The figure shows three views and two pictorial views of one solid part (mm, origin at its lowest corner). Answer the questions. Coordinates: 2 decimals unless noted, no trailing zeros. Write each loop counter-clockwise with the first axis right and the second up, starting at its lowest first coordinate (ties: lowest second). Pieces come first, ordered by that corner, then holes.
Item 1: Section C-C (z = 12.25) is taken. Give the vertices of the cut face in (x, y).
Item 2: Section A-A (y = 0.2) is taken. Give the vertices of the cut face in (x, z), then the cut area to 3 significant figures.
Item 3: Section B-B (x = 8) is taken. Give the vertices of the cut face in (y, z).
Item 4: This flat-tipped pin is pushed along its axis until it touches: P1, Ø3, axis at x = 3, z = 2, coming from the -Y side. Where does it stop, or does it pass through?
Item 5: Straight lines are drawn through the part: probe 1 along X at (y, z) = (0.45, 7.5) (1 decimal); probe 2 along Z at (x, y) = (8, 0.3); probe 3 along Z at (x, y) = (5.5, 0.3). For each, find the intervals that lie inside material, in ascending order.
Item 6: Section D-D (x = 2) is taken. Give the vertices of the cut face in (y, z), then the cut area to 3 significant figures.
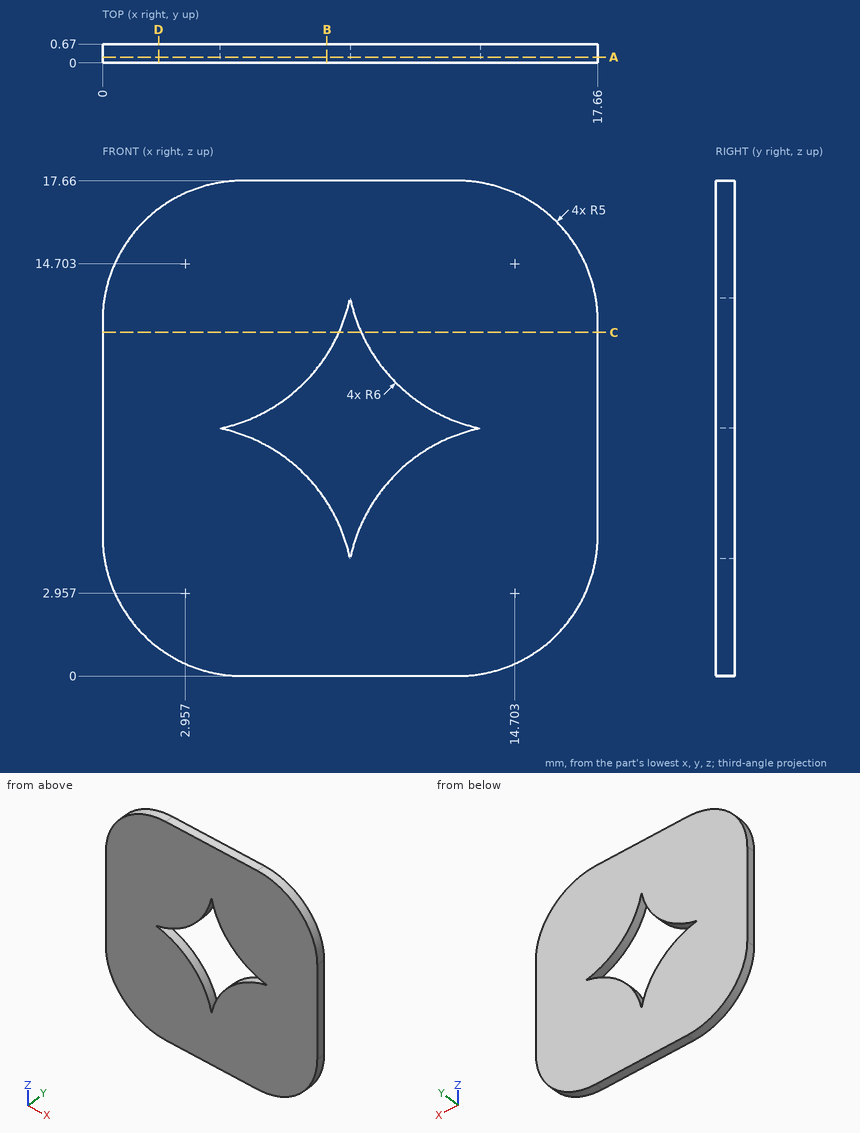
Established:
1. outline: (0, 0) - (8.43, 0) - (8.43, 0.67) - (0, 0.67) - close; (9.23, 0) - (17.66, 0) - (17.66, 0.67) - (9.23, 0.67) - close
2. outline: (0, 5) arc R5 ccw to (5, 0) - (12.66, 0) arc R5 ccw to (17.66, 5) - (17.66, 12.66) arc R5 ccw to (12.66, 17.66) - (5, 17.66) arc R5 ccw to (0, 12.66) - close; hole (4.19, 8.83) arc R6 cw to (8.83, 4.19) arc R6 cw to (13.47, 8.83) arc R6 cw to (8.83, 13.47) arc R6 cw to start
2. area: 265 mm2
3. outline: (0, 0) - (0.67, 0) - (0.67, 6.21) - (0, 6.21) - close; (0, 11.45) - (0.67, 11.45) - (0.67, 17.66) - (0, 17.66) - close
4. P1: stops at y = 0
5. probe 1: x = 0 to 6.9, 10.8 to 17.7
5. probe 2: z = 0 to 6.21, 11.45 to 17.66
5. probe 3: z = 0 to 8.39, 9.27 to 17.66
6. outline: (0, 1) - (0.67, 1) - (0.67, 16.66) - (0, 16.66) - close
6. area: 10.5 mm2
